The listing builds one solid part. Answer for the finished solid, in the listing's coordinates (mm). Give positions to 0.01 mm unless a question says otherwise; leave off trailing zeros.
Item 1: Each of these flat-tipped pins is pushed along its axis until it touches: pin 1 Ø1.5 at (y, z) = (25, 149) entering from +X; pin 2 Ø12 at (x, z) = (-86, 148.5) entering from +Y; pin 3 Ø8 at (x, z) = (-76.5, 145.5) entering from +Y. Where does it stop, or does it pass through?
Item 2: Consider line 1 along Z through (x, y) = (-23.5, 55); line 2 along Y through (x, z) = (-21.5, 143.5); line 3 along Z through (x, y) = (-82.5, 85.5). Determine where each line is inside the solid, lowest interval first.
Item 3: The mould has two halves that part along X. Classify faces 1 (the face through (-39.95, 33.68, 179.51)), 2 (the face through (-5.526, 77, 161)), 3 (the face through (-81, 81, 139.7)): pulls with the +X half, pulls with the -X half, needs draft (parallel to the pull), parting line crosses it, or undercut.
from build123d import *

# Parameters (mm, degrees)
F1_ANGLE = 90


with BuildPart() as f1:
    # F0 (on Front) → F1 (revolve)
    with BuildSketch(Plane.XZ):
        with BuildLine():
            ThreePointArc((-109.985226, 139.7), (-100.982962, 146.33961), (-91.581002, 152.4))
            Line((-91.581002, 152.4), (-103.370511, 152.4))
            Line((-103.370511, 152.4), (-114.3, 152.4))
            ThreePointArc((-114.3, 152.4), (-122.072817, 146.247999), (-129.515096, 139.7))
            Line((-129.515096, 139.7), (-119.979717, 139.7))
            Line((-119.979717, 139.7), (-109.985226, 139.7))
        make_face()
        with BuildLine():
            Line((-114.3, 152.4), (-103.370511, 152.4))
            ThreePointArc((-103.370511, 152.4), (-79.42104, 166.143074), (-53.685891, 176.150639))
            Line((-53.685891, 176.150639), (-53.685891, 182.77876))
            ThreePointArc((-53.685891, 182.77876), (-85.355329, 170.307715), (-114.3, 152.4))
        make_face()
        with BuildLine():
            Line((-103.370511, 152.4), (-91.581002, 152.4))
            ThreePointArc((-91.581002, 152.4), (-61.039594, 166.994036), (-28.285891, 175.535604))
            Line((-28.285891, 175.535604), (-28.285891, 181.964642))
            ThreePointArc((-28.285891, 181.964642), (-41.088854, 179.507461), (-53.685891, 176.150639))
            ThreePointArc((-53.685891, 176.150639), (-79.42104, 166.143074), (-103.370511, 152.4))
        make_face()
    revolve(axis=Axis((-5.526184, 0, 171.786702), (0, 0, -1)), revolution_arc=F1_ANGLE)


solid = f1.part
Worked answers:
1. pin 1: stops at x = -92.31
1. pin 2: stops at y = 91.63
1. pin 3: stops at y = 99.94
2. line 1: z = 166.12 to 179.64
2. line 2: y = 98.16 to 118.7
2. line 3: z = 139.7 to 147.49
3. face 1: undercut
3. face 2: pulls with the +X half
3. face 3: needs draft
